from build123d import *

# Parameters (mm, degrees)
F3_R = 3


# Not quite as in the source:
# - a fillet or chamfer that OpenCascade refuses, or shapes differently, is made with other operations: its cross-section is extruded or revolved along the edge and cut away or added


with BuildPart() as f1:
    # F0 (on Front) → F1 (revolve)
    with BuildSketch(Plane.XZ):
        Polygon((-1, 0), (-1, 20), (-1.75, 20), (-2.5, 17.25), (-2, 17.25), (-2.75, 14.5), (-2.25, 14.5), (-2.25, 3), (-4.6620704234, 3), (-4.6620704234, -3), (-3.5, -3), (-2.8, -23), (-1.6, -23), align=None)
        Polygon((0, -23), (-1.6, -23), (-2.8, -23), (-10, -24.5), (0, -24.5), align=None)
    revolve(axis=Axis((0, 0, 10), (0, 0, 1)))

    # F2: fillet of radius 8 on 2 edges, made by hand

    # F2_s1 → F2_t2 (revolve)
    with BuildSketch(Plane.XZ):
        with BuildLine():
            ThreePointArc((-2.25, 8.7249491741), (-2.8776382138, 5.6187808443), (-4.6620704234, 3))
            Line((-4.6620704234, 3), (-4.5503118318, 2.8855010165))
            ThreePointArc((-4.5503118318, 2.8855010165), (-3.4560352117, 2.84), (-2.25, 2.84))
            Line((-2.25, 2.84), (-2.09, 3))
            Line((-2.09, 3), (-2.09, 8.7249491741))
            Line((-2.09, 8.7249491741), (-2.25, 8.7249491741))
        make_face()
    revolve(axis=Axis((0, 0, 3), (0, 0, 1)))

    # F2_s3 → F2_t4 (revolve)
    with BuildSketch(Plane.XZ):
        with BuildLine():
            ThreePointArc((-4.6620704234, -3), (-3.7272345044, -4.9644393238), (-3.3562164627, -7.1081010661))
            Line((-3.3562164627, -7.1081010661), (-3.1963143727, -7.102504493))
            Line((-3.1963143727, -7.102504493), (-3.3400979101, -2.9944034269))
            Line((-3.3400979101, -2.9944034269), (-3.5, -2.84))
            ThreePointArc((-3.5, -2.84), (-4.0810352117, -2.84), (-4.5282854126, -2.9122414055))
            Line((-4.5282854126, -2.9122414055), (-4.6620704234, -3))
        make_face()
    revolve(axis=Axis((0, 0, -3), (0, 0, 1)))

    # F3
    f3_edges = [f1.edges().sort_by_distance(p)[0] for p in [
        (4.66207, 0, 3),
        (4.66207, 0, -3),
    ]]
    fillet(f3_edges, radius=F3_R)


solid = f1.part
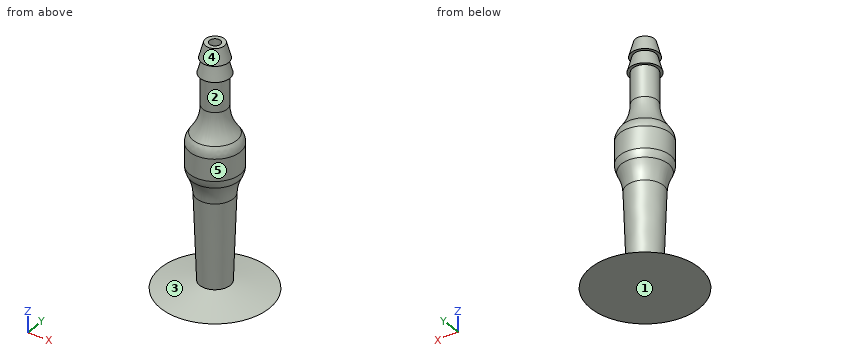
Geometry check sheet. Reference: the model listing, model coordinates, mm. Face numbers are marked on the shaded views. A direction names the side the tool comes from. Round coordinates to 2 decimals unless told otherwise and drop trailing zeros. Loops run counter-clockwise (first coordinate to the right, second up) from the corner with the lowest first, then second, coordinate; pieces in that order, holes last.
Item 1: Mould release check, pull along Z, two halves, no side actions. Record for the marked faces 3, 4 and 5: pulls with the +Z half, pulls with the -Z half, needs draft (parallel to the pull), parting line crosses it, or undercut.
Item 2: Thickness scan on line 1 (Y direction, x = 0, z = 14). Record the ranges inside material, lowest first.
Item 3: Access from +Z, -Z, +X, -X, +Y, -Y to the whole of each face (thin tool, end or side, straight path). Record for the marked faces 1 and 2.
Item 4: Gauge pin test, flat ends, axial feed: pin 1 (1 mm diameter, centred on x = 0, z = -9, fed in from -Y); pin 2 (5 mm diameter, centred on y = -1, z = 4, fed in from +X); pin 3 (8 mm diameter, centred on y = 1, z = -18, fed in from +X); pin 4 (10 mm diameter, centred on x = 5, y = 1.5, fed in from +Z). Record the tip position at first contact, or that the pin passes through.
Item 5: Cross-section at B-B on z = -16. Record the boundary of the cut face in (x, y) (3 decimals).
Item 6: Cross-section at A-A on z = 11. Record the boundary of the cut face in (x, y), then the cut area to 3 significant figures.
Answer sheet:
1. face 3: undercut
1. face 4: pulls with the +Z half
1. face 5: needs draft
2. line 1: y = -2.25 to -1, 1 to 2.25
3. face 1: -Z, +X, -X, +Y, -Y
3. face 2: none
4. pin 1: stops at y = -3.31
4. pin 2: stops at x = 4.66
4. pin 3: stops at x = 3.11
4. pin 4: stops at z = 20
5. outline: circle Ø6.09 at (0, 0); hole circle Ø2.835 at (0, 0)
6. outline: circle Ø4.5 at (0, 0); hole circle Ø2 at (0, 0)
6. area: 12.8 mm2
